Autodesk Inventor part; units mm, degrees
ref_plane "YZ Plane" through (0, 0, 0) normal (1, 0, 0) x (0, 1, 0)
ref_plane "XZ Plane" through (0, 0, 0) normal (0, 1, 0) x (-1, 0, 0)
ref_plane "XY Plane" through (0, 0, 0) normal (0, 0, 1) x (1, 0, 0)
sketch "Boceto1" plane through (0, 0, 0) normal (0, 0, 1) x (1, 0, 0)
  line L0 (-36, 38) -> (36, 38)
  line L1 (38, 36) -> (38, -36)
  line L2 (36, -38) -> (-36, -38)
  line L3 (-38, -36) -> (-38, 36)
  arc A0 (-36, 38) -> (-38, 36) centre (-36, 36) ccw
  arc A1 (38, 36) -> (36, 38) centre (36, 36) ccw
  arc A2 (36, -38) -> (38, -36) centre (36, -36) ccw
  arc A3 (-38, -36) -> (-36, -38) centre (-36, -36) ccw
  line L4 (-36, 36) -> (36, -36) construction
  line L5 (-36, -36) -> (36, 36) construction
  circle A4 centre (23.55, 23.55) radius 2.5
  circle A5 centre (23.55, -23.55) radius 2.5
  circle A6 centre (-23.55, -23.55) radius 2.5
  circle A7 centre (-23.55, 23.55) radius 2.5
  circle A8 centre (0, 0) radius 20
  point P0 (-38, 38)
  point P1 (-38, -38)
  dimension "d0" = 76
  dimension "d1" = 2
  dimension "d2" = 5
  dimension "d3" = 61.6095
  dimension "d4" = 40
  dimension "d23" = 47.1
extrude "Extrusión1" add sketch "Boceto1" against normal blind 8
properties part number "placa soporte motor"
Check sheet for the modelled part. Datum: model origin and axes. Units: mm. Round coordinates to 2 decimals unless told otherwise and drop trailing zeros. Order: outer loops, then holes, each group sorted by start corner. A loop starts at its lowest first (then second) coordinate and runs counter-clockwise, first axis right, second up. Notation, with made-up numbers: M -28.75,-14 L 0.25,-14 A21 ccw 0.25,18 Z; hole C -4,47.5 d5. An arc over 180 degrees is marked long. One line per item, written item: value. Start each with the question number.
1. Gauge pin test, flat end, axial feed: P1, Ø4.5, axis at x = 23.55, y = 23.55, coming from the -Z side. Record the tip position at first contact, or that the pin passes through.
2. Section check C-C on z = -6.25. Enter the section's corners in (x, y), and give its area (3 significant figures).
3. Section check B-B on x = 23.55. Enter the section's corners in (y, z).
4. Release check for a two-part mould opening along X. For faces 1 (the flat face through (-1, 38, -4)), 2 (the cylindrical face through (37.4, -37.43, -3.94)), 3 (the cylindrical face through (-24.09, 21.11, -3.94)) record: released by +X, released by -X, zero draft, split by the parting line, or undercut.
5. Scan lines: line 1 along Y through (x, z) = (-23.55, -6.5); line 2 along Y through (x, z) = (-0.5, -5.5); line 3 along X through (y, z) = (-21.5, -3.5). Record each from-to range of solid material in increasing order.
6. Section check A-A on y = 0. Enter the section's corners in (x, z).
Results found:
1. P1: through
2. outline: M -38,-36 A2 ccw -36,-38 L 36,-38 A2 ccw 38,-36 L 38,36 A2 ccw 36,38 L -36,38 A2 ccw -38,36 Z; hole C -23.55,-23.55 d5; hole C -23.55,23.55 d5; hole C 0,0 d40; hole C 23.55,-23.55 d5; hole C 23.55,23.55 d5
2. area: 4,440 mm^2
3. outline: M -38,-8 L -26.05,-8 L -26.05,0 L -38,0 Z; M -21.05,-8 L 21.05,-8 L 21.05,0 L -21.05,0 Z; M 26.05,-8 L 38,-8 L 38,0 L 26.05,0 Z
4. face 1: zero draft
4. face 2: released by +X
4. face 3: undercut
5. line 1: -38 to -26.05, -21.05 to 21.05, 26.05 to 38
5. line 2: -38 to -19.99, 19.99 to 38
5. line 3: -38 to -24.98, -22.12 to 22.12, 24.98 to 38
6. outline: M -38,-8 L -20,-8 L -20,0 L -38,0 Z; M 20,-8 L 38,-8 L 38,0 L 20,0 Z
